from build123d import *

# Parameters (mm, degrees)
SKETCH018_W             = 40
SKETCH018_H             = 43
PAD013_DEPTH            = 3
SKETCH019_R             = 1.5
PAD014_DEPTH            = 3
SKETCH020_R             = 2
POCKET003_DEPTH         = 3.001
FILLET_R                = 1
POCKET004_DEPTH         = 40.001
BODY001_PLACEMENT_ANGLE = 90


with BuildPart() as part:
    # Sketch018 → Pad013 (new body)
    with BuildSketch(Plane.XY):
        Rectangle(SKETCH018_W, SKETCH018_H)
    extrude(amount=PAD013_DEPTH)

    # Sketch019 (on Face1 of Pad013) → Pad014 (join)
    with BuildSketch(Plane(origin=(0, 21.5, 0), x_dir=(-1, 0, 0), z_dir=(0, 1, 0))):
        with BuildLine():
            Line((-20, 3), (20, 3))
            Line((20, 3), (20, 27))
            ThreePointArc((20, 27), (0, 47), (-20, 27))
            Line((-20, 27), (-20, 3))
        make_face()
        with Locations((-7.75, 40.42)):
            Circle(SKETCH019_R, mode=Mode.SUBTRACT)
        with Locations((7.75, 40.42)):
            Circle(SKETCH019_R, mode=Mode.SUBTRACT)
        with Locations((15.5, 27)):
            Circle(SKETCH019_R, mode=Mode.SUBTRACT)
        with Locations((-15.5, 27)):
            Circle(SKETCH019_R, mode=Mode.SUBTRACT)
        with Locations((-7.75, 13.58)):
            Circle(SKETCH019_R, mode=Mode.SUBTRACT)
        with Locations((7.75, 13.58)):
            Circle(SKETCH019_R, mode=Mode.SUBTRACT)
        with BuildLine():
            ThreePointArc((6.5, 34), (0, 40.5), (-6.5, 34))
            Line((-6.5, 34), (-6.5, 20))
            ThreePointArc((-6.5, 20), (0, 13.5), (6.5, 20))
            Line((6.5, 20), (6.5, 34))
        make_face(mode=Mode.SUBTRACT)
    extrude(amount=-PAD014_DEPTH)

    # Sketch020 (on Face7 of Pad014) → Pocket003 (cut, through all)
    with BuildSketch(Plane.XY.offset(3)):
        with Locations((15, 10.5)):
            Circle(SKETCH020_R)
        with Locations((15, -13.5)):
            Circle(SKETCH020_R)
        with Locations((-15, 10.5)):
            Circle(SKETCH020_R)
        with Locations((-15, -13.5)):
            Circle(SKETCH020_R)
    extrude(amount=-POCKET003_DEPTH, mode=Mode.SUBTRACT)

    # Fillet
    fillet_edges = [part.edges().sort_by_distance(p)[0] for p in [
        (0, 18.5, 3),
    ]]
    fillet(fillet_edges, radius=FILLET_R)

    # Sketch021 (on Face1 of Fillet) → Pocket004 (cut, through all)
    with BuildSketch(Plane(origin=(-20, 0, 0), x_dir=(0, -1, 0), z_dir=(-1, 0, 0))):
        with BuildLine():
            ThreePointArc((-21.5, 3), (-20.415476, 1.084524), (-18.5, 0))
            Line((-21.5, 0), (-18.5, 0))
            Line((-21.5, 3), (-21.5, 0))
        make_face()
    extrude(amount=-POCKET004_DEPTH, mode=Mode.SUBTRACT)


with BuildPart() as part_1:
    # Body001 placement: moved
    add(part.part.moved(Location((445.5, -85, 0))).rotate(Axis((445.5, -85, 0), (0, 1, 0)), BODY001_PLACEMENT_ANGLE))


solid = part_1.part
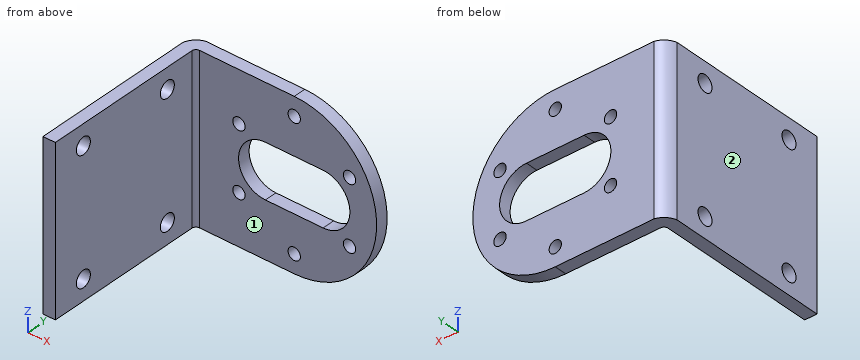
The model under review builds one solid part; all positions refer to its coordinate system, in mm. Face numbers are marked on the shaded views. A direction names the side the tool comes from. Round coordinates to 2 decimals unless told otherwise and drop trailing zeros. Loops run counter-clockwise (first coordinate to the right, second up) from the corner with the lowest first, then second, coordinate; pieces in that order, holes last. Notation, with made-up numbers: M 67.25,-32.75 L 121.25,-32.75 A24 cw 121.25,2.25 Z; hole C 83.25,-10 d3. An arc over 180 degrees is marked long. Answer as a JSON object with one key per item and string values.
Item 1: For line 1 along Z through (x, y) = (446.3, -74.5); line 2 along Z through (x, y) = (447, -98); line 3 along X through (y, z) = (-65.1, 7.75), list the stretches that pass through material, from the lowest coordinate up.
Check sheet entries:
{"line 1": "-20 to -17, -13 to 13, 17 to 20", "line 2": "-20 to -16.94, -13.06 to 13.06, 16.94 to 20", "line 3": "446.15 to 457.58, 460.58 to 484.42, 487.42 to 490.94"}
Item 2: Tool access review of the marked faces 1 and 2: name each direction out of +Z, -Z, +X, -X, +Y, -Y from which nothing blocks a thin tool from reaching the whole face with its end or side.
Check sheet entries:
{"face 1": "+Z, -Z, +X, -Y", "face 2": "+Z, -Z, -X, +Y, -Y"}
Item 3: We need section B-B, the plane z = 7.75. State the section outline as (x, y) points, and give its area (3 significant figures).
Check sheet entries:
{"outline": "M 445.5,-106.5 L 448.5,-106.5 L 448.5,-67.5 A1 cw 449.5,-66.5 L 457.58,-66.5 L 457.58,-63.5 L 448.5,-63.5 A4.12 ccw 445.5,-66.5 Z; M 460.58,-66.5 L 484.42,-66.5 L 484.42,-63.5 L 460.58,-63.5 Z; M 487.42,-66.5 L 490.94,-66.5 L 490.94,-63.5 L 487.42,-63.5 Z", "area": "236 mm2"}
Item 4: We need section D-D, the plane x = 454. State the section outline as (y, z) points, and give its area (3 significant figures).
Check sheet entries:
{"outline": "M -66.5,-20 L -63.5,-20 L -63.5,20 L -66.5,20 Z", "area": "120 mm2"}
Item 5: Clearance check with flat-ended pins moving along their axes: P1, Ø2.5, axis at x = 459.08, z = -7.75, coming from the +Y side; P2, Ø4, axis at y = -79, z = -9.5, coming from the +X side; P3, Ø20, axis at x = 480.5, z = 3, coming from the -Y side. State where each tip first meets the part, or that it passes through.
Check sheet entries:
{"P1": "through", "P2": "x = 448.5", "P3": "y = -66.5"}
Item 6: We need section A-A, the plane y = -98.5. State the section outline as (x, z) points.
Check sheet entries:
{"outline": "M 445.5,-20 L 448.5,-20 L 448.5,-17 L 445.5,-17 Z; M 445.5,-13 L 448.5,-13 L 448.5,13 L 445.5,13 Z; M 445.5,17 L 448.5,17 L 448.5,20 L 445.5,20 Z"}
Item 7: We need section C-C, the plane z = 15. State the section outline as (x, y) points, and give its area (3 significant figures).
Check sheet entries:
{"outline": "M 445.5,-106.5 L 448.5,-106.5 L 448.5,-100.5 L 445.5,-100.5 Z; M 445.5,-96.5 L 448.5,-96.5 L 448.5,-76.5 L 445.5,-76.5 Z; M 445.5,-72.5 L 448.5,-72.5 L 448.5,-67.5 A1 cw 449.5,-66.5 L 471.09,-66.5 L 471.09,-63.5 L 448.5,-63.5 A4.12 ccw 445.5,-66.5 Z; M 473.91,-66.5 L 485.73,-66.5 L 485.73,-63.5 L 473.91,-63.5 Z", "area": "206 mm2"}
